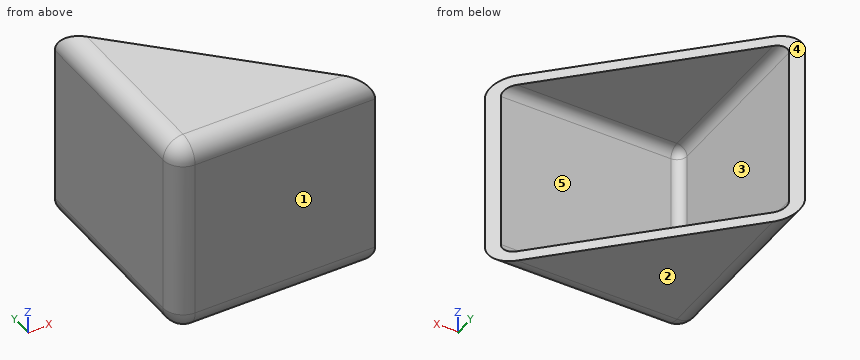
```python
from build123d import *

# Parameters (mm, degrees)
F1_DEPTH = 50
F2_R     = 5
F3_T     = -2.5


with BuildPart() as f1:
    # F0 (on Top) → F1 (new body)
    with BuildSketch(Plane.XY):
        Polygon((-4.141866, 45.817343), (-4.141866, -4.182657), (45.858134, -4.182657), align=None)
    extrude(amount=F1_DEPTH)

    # F2
    f2_edges = [f1.edges().sort_by_distance(p)[0] for p in [
        (-4.141866, -4.182657, 25),
        (20.858134, -4.182657, 0),
        (-4.141866, 20.817343, 0),
        (-4.141866, 20.817343, 50),
        (20.858134, -4.182657, 50),
    ]]
    fillet(f2_edges, radius=F2_R)

    # F3
    f3_openings = [f1.faces().sort_by_distance(p)[0] for p in [
        (20.858134, 20.817343, 25),
    ]]
    offset(amount=F3_T, openings=f3_openings)


solid = f1.part
```
For this review, take the finished solid that the model builds, in its own axes (mm). Face numbers are marked on the shaded views. A direction names the side the tool comes from. Give positions to 0.01 mm unless a question says otherwise; leave off trailing zeros. Write each loop counter-clockwise with the first axis right and the second up, starting at its lowest first coordinate (ties: lowest second). Pieces come first, ordered by that corner, then holes.
Item 1: The part is to be moulded in two halves that separate along Z. For the marked faces 1, 2 and 3, say which applies: +Z half, -Z half, draft (parallel to the pull), parting line (faces both ways), or undercut.
Item 2: Take a section at B-B (y = 30.5). Give the boundary of the cut face in (x, z), and give its area (3 significant figures).
Item 3: Take a section at C-C (x = 13.5). Give the boundary of the cut face in (y, z), and give its area (3 significant figures).
Item 4: Wall thickness on probe 1 along Z at (x, y) = (25.5, 6.5); probe 2 along X at (y, z) = (35, 38.5); probe 3 along Y at (x, z) = (41.5, 17): over which ranges is each line inside the solid? List them lowest first.
Item 5: Insertion check: P1, Ø3, axis at x = 4.5, z = 30.5, coming from the +Y side. The pin has a flat end and moves straight along its axis. Give the tip position at first contact, or say it passes through.
Item 6: Take a section at A-A (z = 43). Give the boundary of the cut face in (x, y), and give its area (3 significant figures).
Item 7: Machinability: for the marked faces 4 and 5, which of the approach directions +Z, -Z, +X, -X, +Y, -Y give a long, thin tool a straight path to every point of the face, cutting with its end or side? Answer none if there is none.
Established:
1. face 1: draft
1. face 2: -Z half
1. face 3: undercut
2. outline: (-4.14, 5) arc R5 ccw to (0.86, 0) - (11.18, 0) - (11.18, 2.5) - (0.86, 2.5) arc R2.5 cw to (-1.64, 5) - (-1.64, 45) arc R2.5 cw to (0.86, 47.5) - (11.18, 47.5) - (11.18, 50) - (0.86, 50) arc R5 ccw to (-4.14, 45) - close
2. area: 181 mm2
3. outline: (-4.18, 5) arc R5 ccw to (0.82, 0) - (28.18, 0) - (28.18, 2.5) - (0.82, 2.5) arc R2.5 cw to (-1.68, 5) - (-1.68, 45) arc R2.5 cw to (0.82, 47.5) - (28.18, 47.5) - (28.18, 50) - (0.82, 50) arc R5 ccw to (-4.18, 45) - close
3. area: 266 mm2
4. probe 1: z = 0 to 2.5, 47.5 to 50
4. probe 2: x = -4.14 to -1.64
4. probe 3: y = -4.18 to -1.68
5. P1: stops at y = -1.68
6. outline: (-4.14, 0.82) arc R5 ccw to (0.86, -4.18) - (45.86, -4.18) - (43.36, -1.68) - (0.86, -1.68) arc R2.5 cw to (-1.64, 0.82) - (-1.64, 43.32) - (-4.14, 45.82) - close
6. area: 233 mm2
7. face 4: +Z, -Z, +X, +Y
7. face 5: +X, +Y
